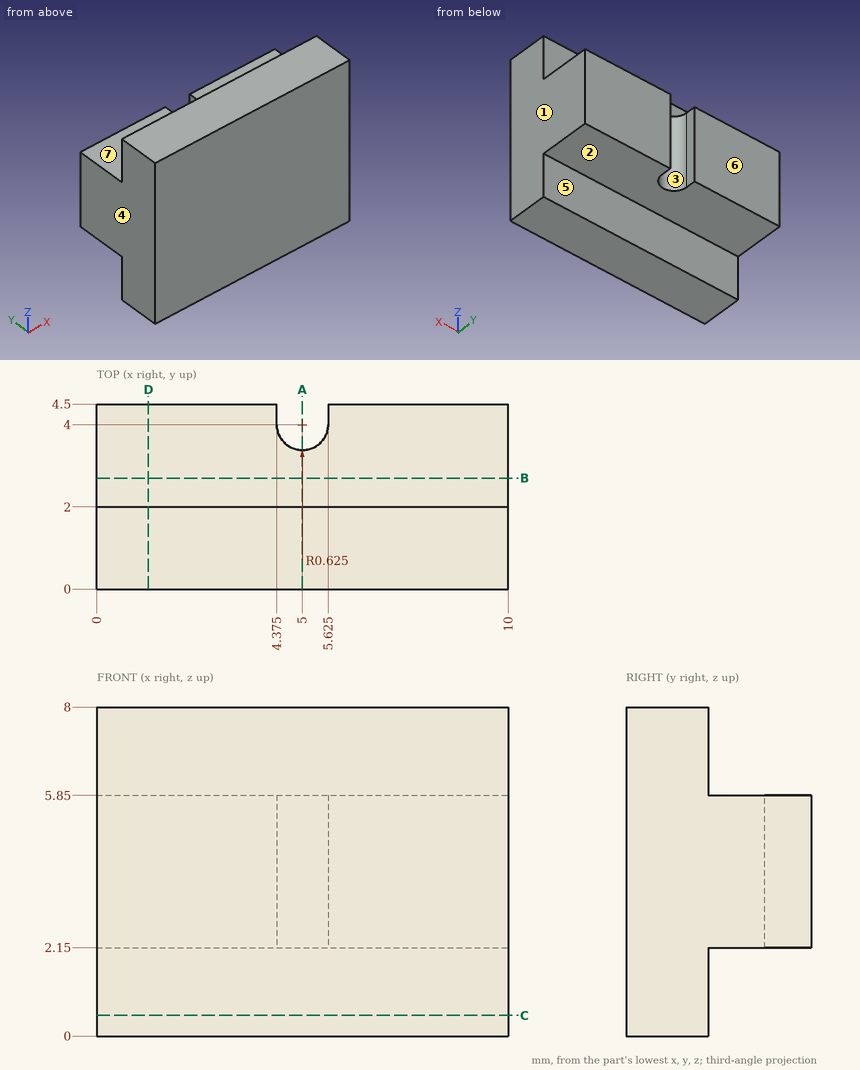
Geometry: see drawing. Coordinates: mm, zero at the bounding-box minimum. A direction names the side the tool comes from. Coordinates: 2 decimals unless noted, no trailing zeros. Loops run counter-clockwise (first coordinate to the right, second up) from the corner with the lowest first, then second, coordinate; pieces in that order, holes last. Notation, with made-up numbers: M 27.25,53.5 L 38.25,53.5 A14 ccw 38.25,61.5 Z; hole C -25.75,30.25 d1. An arc over 180 degrees is marked long. Answer in a Markdown table with one row per item.
Q1. Section A-A on x = 5. Return the cut outline in (y, z) (3 decimals).
Answers below:
| item | result |
|---|---|
| outline | M 0,0 L 2,0 L 2,2.15 L 3.375,2.15 L 3.375,5.85 L 2,5.85 L 2,8 L 0,8 Z |
Q2. Ray query, probe 1 along X at (y, z) = (4, 4.75) (3 decimals); probe 2 along Y at (x, z) = (5.25, 6.75); probe 3 along Z at (x, y) = (1.25, 3.7). Return the intervals inside material, ascending. Write a range as from..to.
Answers below:
| item | result |
|---|---|
| probe 1 | x = 0..4.375, 5.625..10 |
| probe 2 | y = 0..2 |
| probe 3 | z = 2.15..5.85 |
Q3. Section C-C on z = 0.5. Return the cut outline in (x, y), plus the area to 3 significant figures.
Answers below:
| item | result |
|---|---|
| outline | M 0,0 L 10,0 L 10,2 L 0,2 Z |
| area | 20.0 mm^2 |
Q4. First-contact query: pin 1 (1.7 mm diameter, centred on x = 7, z = 1, fed in from +Y); pin 2 (1.5 mm diameter, centred on x = 3.5, y = 4, fed in from +Z). Flat tips, straight axial feed; report the tip coordinate or a pass-through.
Answers below:
| item | result |
|---|---|
| pin 1 | stops at y = 2 |
| pin 2 | stops at z = 5.85 |
Q5. Section D-D on x = 1.25. Return the cut outline in (y, z).
Answers below:
| item | result |
|---|---|
| outline | M 0,0 L 2,0 L 2,2.15 L 4.5,2.15 L 4.5,5.85 L 2,5.85 L 2,8 L 0,8 Z |
Q6. Draft query along X for the marked faces 1, 2, 3 and 4. Return one class per face: pulls with the +X half, pulls with the -X half, needs draft (parallel to the pull), parting line crosses it, or undercut.
Answers below:
| item | result |
|---|---|
| face 1 | pulls with the +X half |
| face 2 | needs draft |
| face 3 | undercut |
| face 4 | pulls with the -X half |
Q7. Set-up query: the marked faces 5, 6 and 7. Return all of +Z, -Z, +X, -X, +Y, -Y with unobstructed straight access to the full face (end or side cutting, diameter ignored); none if empty.
Answers below:
| item | result |
|---|---|
| face 5 | -Z, +X, -X, +Y |
| face 6 | +Z, -Z, +X, -X, +Y |
| face 7 | +Z, +X, -X, +Y |
Q8. Section B-B on y = 2.7. Return the cut outline in (x, z), plus the area to 3 significant figures.
Answers below:
| item | result |
|---|---|
| outline | M 0,2.15 L 10,2.15 L 10,5.85 L 0,5.85 Z |
| area | 37.0 mm^2 |
